from build123d import *

# Parameters (mm, degrees)
F0_R        = 1.75
F1_DEPTH    = 5
F2_DEPTH    = 9
F3_T1_DEPTH = 31.689764736
F4_R        = 9.8818743841


# Not quite as in the source:
# - a fillet or chamfer that OpenCascade refuses, or shapes differently, is made with other operations: its cross-section is extruded or revolved along the edge and cut away or added


with BuildPart() as f1:
    # F0 (on Top) → F1 (new body)
    with BuildSketch(Plane.XY):
        with BuildLine():
            ThreePointArc((10.3788942671, 7.8619225196), (14.645060229, 7.8336341982), (16.7863510811, 11.523599744))
            ThreePointArc((16.7863510811, 11.523599744), (12.5363510811, 15.773599744), (8.2863510811, 11.523599744))
            ThreePointArc((8.2863510811, 11.523599744), (8.8463855352, 9.4148905962), (10.3788942671, 7.8619225196))
        make_face()
        with Locations((12.5363510811, 11.523599744)):
            Circle(F0_R, mode=Mode.SUBTRACT)
        with BuildLine():
            ThreePointArc((10.3788942671, 7.8619225196), (8.8463855352, 9.4148905962), (8.2863510811, 11.523599744))
            Line((8.2863510811, 11.523599744), (-8.3690416068, -7.120377686))
            Line((-8.3690416068, -7.120377686), (-5.386005218, -9.7852405161))
            Line((-5.386005218, -9.7852405161), (10.3788942671, 7.8619225196))
        make_face()
        Polygon((-5.386005218, -9.7852405161), (-8.3690416068, -7.120377686), (-8.3690416068, -9.7852405161), align=None)
    extrude(amount=F1_DEPTH)

    # F0 (on Top) → F2 (join)
    with BuildSketch(Plane.XY):
        with Locations((12.5363510811, 11.523599744)):
            Circle(F0_R)
    extrude(amount=F2_DEPTH)

    # F3: fillet of radius 16 on 1 edges, made by hand

    # F3_s2 → F3_t1 (cut)
    with BuildSketch(Plane.XY.offset(-13.344882368)):
        with BuildLine():
            ThreePointArc((-4.8128135074, -3.1395507152), (-6.9878475663, -6.2499965822), (-8.3690416068, -9.7852405161))
            Line((-8.3690416068, -9.7852405161), (-8.3690416068, -7.120377686))
            Line((-8.3690416068, -7.120377686), (-4.8128135074, -3.1395507152))
        make_face()
    extrude(amount=F3_T1_DEPTH, mode=Mode.SUBTRACT)

    # F4
    f4_edges = [f1.edges().sort_by_distance(p)[0] for p in [
        (8.286351, 11.5236, 2.5),
        (10.378894, 7.861923, 2.5),
    ]]
    fillet(f4_edges, radius=F4_R)


solid = f1.part
Geometry check sheet. Reference: the model listing, model coordinates, mm. A direction names the side the tool comes from. Coordinates: 2 decimals unless noted, no trailing zeros. Order: outer loops, then holes, each group sorted by start corner. A loop starts at its lowest first (then second) coordinate and runs counter-clockwise, first axis right, second up. Notation, with made-up numbers: (-11, 46.25) -> (0, 46.25) arc R16 ccw to (0, 72.25) -> close; hole circle Ø7 at (-37.75, -21.5). An arc over 180 degrees is marked (long way). Use a Markdown table: item, result. Add a question column.
1. Cross-section at D-D (z = 6.25). Enter the section's corners in (x, y), and give its area (3 significant figures).
2. Cross-section at C-C (y = -2.25). Enter the section's corners in (x, z).
3. Cross-section at B-B (x = 2.5). Enter the section's corners in (y, z).
4. Material ranges on L1, parallel to Z at x = 12.25, y = 8.5; L2, parallel to X at y = -2.75, z = 2.5; L3, parallel to X at y = 11.5, z = 2, recorded low to high.
5. Set-up check for faces 1 (the face through (0.954, 3.316, 2.465)), 2 (the face through (12.31, 13.26, 6.97)): record each of +Z, -Z, +X, -X, +Y, -Y from which the full face is reachable in a straight line by a thin tool's end or side.
6. Go/stop test with flat-tipped pins: pin 1 Ø1 at (x, y) = (-1.5, -6.5) entering from +Z; pin 2 Ø4 at (y, z) = (12, 1) entering from -X; pin 3 Ø4 at (x, z) = (-4.5, 5.5) entering from +Y; pin 4 Ø1 at (x, z) = (5, 2.5) entering from +Y. Record where each tip stops, or that it passes through.
7. Cross-section at A-A (z = 3.5). Enter the section's corners in (x, y), and give its area (3 significant figures).
Filled sheet:
| question | item | result |
|---|---|---|
| 1 | outline | circle Ø3.5 at (12.54, 11.52) |
| 1 | area | 9.62 mm2 |
| 2 | outline | (-4.02, 0) -> (1.35, 0) -> (1.35, 5) -> (-4.02, 5) -> close |
| 3 | outline | (-0.96, 0) -> (5.05, 0) -> (5.05, 5) -> (-0.96, 5) -> close |
| 4 | L1 | 0 to 5 |
| 4 | L2 | -4.46 to 0.9 |
| 4 | L3 | 7.9 to 16.79 |
| 5 | face 1 | +Z, -Z, -X, +Y |
| 5 | face 2 | +Z |
| 6 | pin 1 | through |
| 6 | pin 2 | x = 6.91 |
| 6 | pin 3 | y = -0.62 |
| 6 | pin 4 | y = 8.4 |
| 7 | outline | (-8.37, -9.79) -> (-5.39, -9.79) -> (7.02, 4.1) arc R9.88 cw to (13.09, 7.31) arc R4.25 ccw (long way) to (8.52, 12.92) arc R9.88 cw to (6.56, 9.59) -> (-4.81, -3.14) arc R16 ccw to start |
| 7 | area | 157 mm2 |
